Autodesk Inventor part; units mm, degrees
ref_plane "YZ Plane" through (0, 0, 0) normal (1, 0, 0) x (0, 1, 0)
ref_plane "XZ Plane" through (0, 0, 0) normal (0, 1, 0) x (-1, 0, 0)
ref_plane "XY Plane" through (0, 0, 0) normal (0, 0, 1) x (1, 0, 0)
sketch "Sketch1" plane through (0, 0, 0) normal (0, 0, 1) x (1, 0, 0)
  line L0 (24.765, -64.933) -> (24.765, -65.405)
  line L1 (41.91, -65.405) -> (24.765, -65.405)
  line L2 (41.91, 0) -> (41.91, -65.405)
  line L3 (0, 0) -> (41.91, 0)
  line L4 (0, -65.405) -> (0, 0)
  line L5 (17.145, -65.405) -> (0, -65.405)
  line L6 (17.145, -65.405) -> (17.145, -64.933)
  line L7 (17.145, -64.933) -> (0.472, -64.933)
  line L8 (0.472, -64.933) -> (0.472, -0.472)
  line L9 (0.472, -0.472) -> (41.438, -0.472)
  line L10 (41.438, -0.472) -> (41.438, -64.933)
  line L11 (41.438, -64.933) -> (24.765, -64.933)
  line L12 (17.145, -64.933) -> (17.145, -63.6597)
  line L13 (17.145, -63.6597) -> (3.0153, -63.6597)
  arc A0 (1.7453, -62.3897) -> (3.0153, -63.6597) centre (3.0153, -62.3897) ccw
  line L14 (1.7453, -62.3897) -> (1.7453, -10.7786)
  arc A1 (1.7453, -10.7786) -> (0.472, -9.5086) centre (0.4753, -10.7786) ccw
  line L15 (0.472, -64.933) -> (0.472, -9.5086)
  line L16 (17.145, -64.933) -> (0.472, -64.933)
  line L17 (24.765, -63.6597) -> (24.765, -64.933)
  line L18 (41.438, -64.933) -> (24.765, -64.933)
  line L19 (41.438, -9.5086) -> (41.438, -64.933)
  arc A2 (41.438, -9.5086) -> (40.1647, -10.7786) centre (41.4347, -10.7786) ccw
  line L20 (40.1647, -10.7786) -> (40.1647, -62.3897)
  arc A3 (38.8947, -63.6597) -> (40.1647, -62.3897) centre (38.8947, -62.3897) ccw
  line L21 (38.8947, -63.6597) -> (24.765, -63.6597)
  line L22 (24.765, -67.945) -> (17.145, -67.945)
  line L23 (24.765, -63.6597) -> (24.765, -67.945)
  line L24 (17.145, -63.6597) -> (24.765, -63.6597)
  line L25 (17.145, -67.945) -> (17.145, -63.6597)
  point P0 (4.318, 23.368)
extrude "Extrusion1" add sketch "Sketch1" along normal blind 1.7526 contours L17 L21 A3 L20 A2 L10 L11 | L0 L23 L22 L25 L6 L12 L24 L17 | L24 L13 A0 L14 A1 L8 L9 L10 A2 L20 A3 L21 | L12 L7 L8 A1 L14 A0 L13
sketch "Sketch2" plane through (0, 0, 0) normal (0, 0, -1) x (-1, 0, 0)
  line L0 (-41.438, -0.472) -> (-0.472, -0.472)
  line L1 (-41.438, -64.933) -> (-41.438, -0.472)
  line L2 (-24.765, -64.933) -> (-41.438, -64.933)
  line L3 (-24.765, -67.945) -> (-24.765, -64.933)
  line L4 (-17.145, -67.945) -> (-24.765, -67.945)
  line L5 (-17.145, -64.933) -> (-17.145, -67.945)
  line L6 (-0.472, -64.933) -> (-17.145, -64.933)
  line L7 (-0.472, -0.472) -> (-0.472, -64.933)
  line L8 (-39.914, -61.885) -> (-39.914, -0.472)
  line L9 (-1.996, -0.472) -> (-1.996, -61.885)
  line L10 (-3.52, -63.409) -> (-38.39, -63.409)
  arc A0 (-39.914, -61.885) -> (-38.39, -63.409) centre (-38.39, -61.885) ccw
  arc A1 (-3.52, -63.409) -> (-1.996, -61.885) centre (-3.52, -61.885) ccw
  line L11 (-41.438, -0.472) -> (-0.472, -0.472)
  line L12 (-4.536, 2.068) -> (-37.374, 2.068)
  line L13 (-1.996, -0.472) -> (-1.996, -0.472)
  line L14 (-37.374, 2.068) -> (-39.914, -0.472)
  line L15 (-4.536, 2.068) -> (-1.996, -0.472)
  point P0 (0, 0)
  point P1 (-39.914, 2.068)
  point P2 (-1.996, 2.068)
  dimension "d2" = 1.524
  dimension "d3" = 1.524
  dimension "d4" = 1.524
  dimension "d5" = 1.524
  dimension "d7" = 2.54
  dimension "d8" = 2.54
  dimension "d9" = 2.54
  dimension "d10" = 2.54
extrude "Extrusion2" add sketch "Sketch2" along normal blind 1.27 contours L14 L12 L15 L0 | L0 L9 A1 L10 A0 L8
chamfer "Chamfer1" distance 1.27 angle 45 1 edges at (20.955, -67.945, 0)
sketch "Sketch3" plane through (0, 0, 1.7526) normal (0, 0, 1) x (1, 0, 0)
  line L0 (41.438, -0.472) -> (0.472, -0.472)
  line L1 (0.472, -0.472) -> (0.472, -64.933)
  line L2 (0.472, -64.933) -> (17.145, -64.933)
  line L3 (17.145, -64.933) -> (17.145, -67.945)
  line L4 (17.145, -67.945) -> (24.765, -67.945)
  line L5 (24.765, -67.945) -> (24.765, -64.933)
  line L6 (24.765, -64.933) -> (41.438, -64.933)
  line L7 (41.438, -64.933) -> (41.438, -0.472)
  line L8 (41.063, -0.847) -> (0.847, -0.847)
  line L9 (0.847, -0.847) -> (0.847, -64.558)
  line L10 (0.847, -64.558) -> (17.52, -64.558)
  line L11 (17.52, -64.558) -> (17.52, -67.57)
  line L12 (17.52, -67.57) -> (24.39, -67.57)
  line L13 (24.39, -67.57) -> (24.39, -64.558)
  line L14 (24.39, -64.558) -> (41.063, -64.558)
  line L15 (41.063, -64.558) -> (41.063, -0.847)
  point P0 (0, 0)
extrude "Extrusion3" cut sketch "Sketch3" against normal up to surface (1.7526 mm away)
sketch "Sketch4" plane through (0, 0, 0) normal (0, 0, 1) x (1, 0, 0)
  line L0 (37.374, 2.068) -> (39.914, -0.472)
  line L1 (4.536, 2.068) -> (37.374, 2.068)
  line L2 (1.996, -0.472) -> (4.536, 2.068)
  line L3 (1.996, -0.472) -> (1.996, -0.847)
  line L4 (1.996, -0.847) -> (39.914, -0.847)
  line L5 (39.914, -0.847) -> (39.914, -0.472)
  line L6 (1.996, -0.472) -> (4.536, 2.068)
  line L7 (3.266, 0.798) -> (38.644, 0.798)
  line L8 (38.644, 0.798) -> (38.644, 2.068)
  line L9 (38.644, 2.068) -> (3.266, 2.068)
  line L10 (3.266, 2.068) -> (3.266, 0.798)
  point P0 (0, 0)
extrude "Extrusion4" cut sketch "Sketch4" against normal blind 1.27 contours L9 L8 L0 | L0 L7 L2 L1 | L2 L10 L9
properties part number "Main_Housing_Cap"
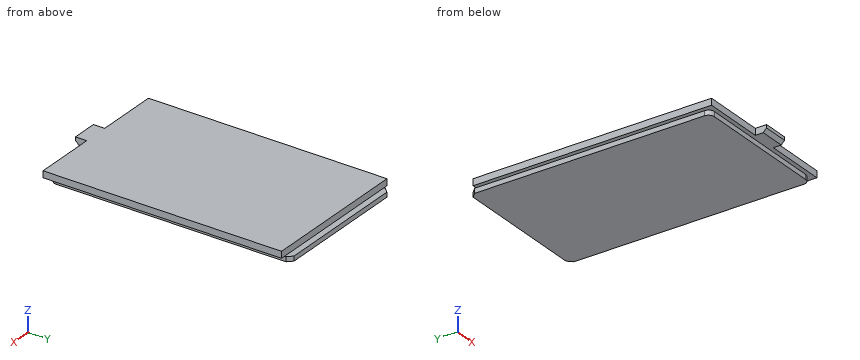
Work out the finished part from the listing and answer in its coordinate system (mm). Give positions to 0.01 mm unless a question says otherwise; leave off trailing zeros. Order: outer loops, then holes, each group sorted by start corner. A loop starts at its lowest first (then second) coordinate and runs counter-clockwise, first axis right, second up. Notation, with made-up numbers: M 87.25,66.5 L 110.25,66.5 A26 ccw 110.25,88.5 Z; hole C 19.5,53.25 d8. An arc over 180 degrees is marked long. Return JSON: item names as keys, results as strings.
Q1. Each of these flat-tipped pins is pushed along its axis until it touches: pin 1 (0.8 mm diameter, centred on x = 20, y = 0, fed in from +Z); pin 2 (1.4 mm diameter, centred on x = 12.5, z = 0.5, fed in from -Y); pin 3 (1.4 mm diameter, centred on y = -66, z = 1.5, fed in from -X). Where does it stop, or does it pass through?
Answer below:
{"pin 1": "stops at z = 0", "pin 2": "stops at y = -64.56", "pin 3": "stops at x = 17.52"}
Q2. Find section B-B, the plane y = -48.5. Write down the section's boundary in (x, z).
Answer below:
{"outline": "M 0.85,0 L 2,0 L 2,-1.27 L 39.91,-1.27 L 39.91,0 L 41.06,0 L 41.06,1.75 L 0.85,1.75 Z"}
Q3. Find the intervals of material crossed by line 1 along Y through (x, z) = (6.5, 0.6); line 2 along Y through (x, z) = (15.5, -1); line 3 along X through (y, z) = (-14.5, -0.2), in increasing order. Write a range as [from, to].
Answer below:
{"line 1": "y = [-64.56, -0.85]", "line 2": "y = [-63.41, 0.8]", "line 3": "x = [2, 39.91]"}
Q4. Find section A-A, the plane x = 21.5. Write down the section's boundary in (y, z) (3 decimals), and give its area (3 significant figures).
Answer below:
{"outline": "M -67.57,0.895 L -66.675,0 L -63.409,0 L -63.409,-1.27 L 0.798,-1.27 L 0.798,0 L -0.847,0 L -0.847,1.753 L -67.57,1.753 Z", "area": "198 mm^2"}
Q5. Find section C-C, the plane z = -0.8. Write down the section's boundary in (x, y) (3 decimals).
Answer below:
{"outline": "M 1.996,-61.885 A1.524 ccw 3.52,-63.409 L 38.39,-63.409 A1.524 ccw 39.914,-61.885 L 39.914,-0.472 L 38.644,0.798 L 3.266,0.798 L 1.996,-0.472 Z"}
